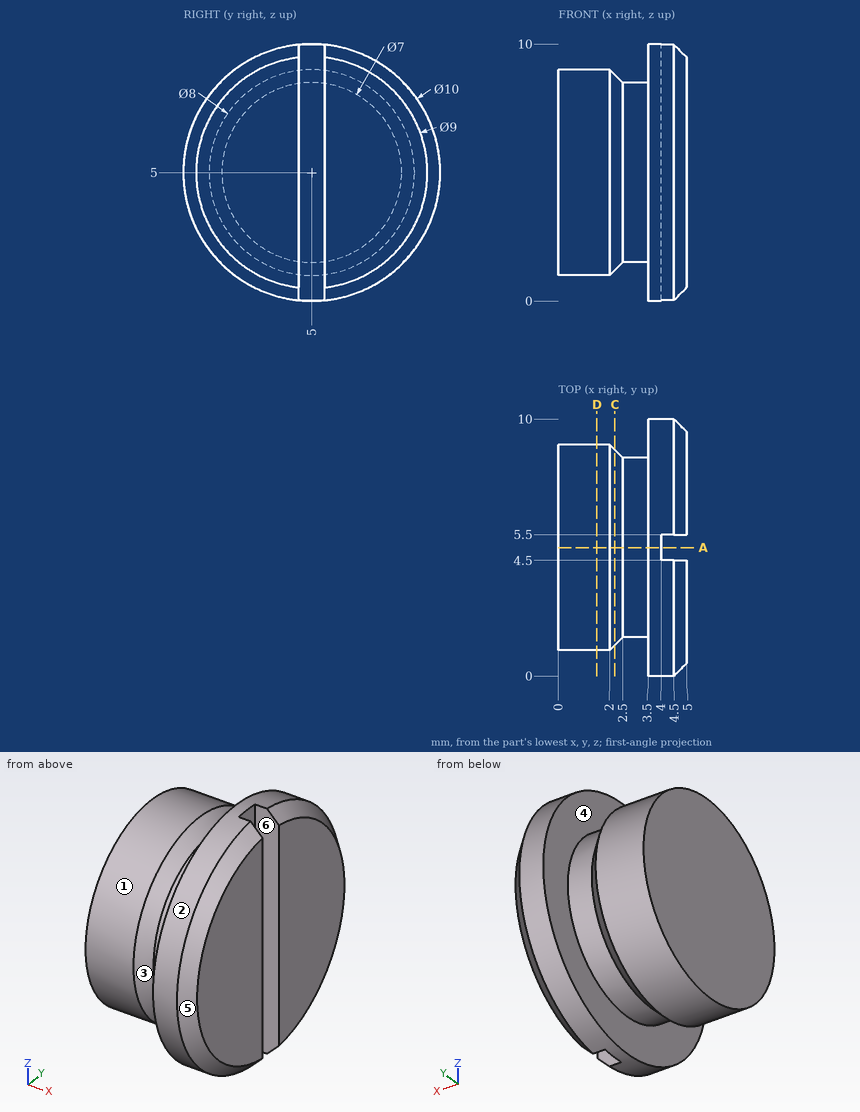
Drawing for the job (mm, zero at the part's lowest x, y, z). A direction names the side the tool comes from. Coordinates: 2 decimals unless noted, no trailing zeros. Order: outer loops, then holes, each group sorted by start corner. A loop starts at its lowest first (then second) coordinate and runs counter-clockwise, first axis right, second up. Notation, with made-up numbers: (-1.75, -33.5) -> (22.25, -33.5) arc R14 ccw to (22.25, -8.5) -> close; hole circle Ø10 at (54.5, 53.25). An arc over 180 degrees is marked (long way). Answer in a Markdown table with one row per item.
1) Band-saw the part on C-C (x = 2.2). List the corners of the cut face in (y, z), and give its area (3 significant figures).
Check values:
| item | result |
|---|---|
| outline | circle Ø7.6 at (5, 5) |
| area | 45.4 mm2 |
2) Flat gauge pins, fed straight in: P1, Ø1.1, axis at x = 4.5, z = 2.5, coming from the -Y side; P2, Ø1.5, axis at x = 2.5, z = 7.5, coming from the -Y side; P3, Ø2, axis at x = 2, y = 5, coming from the -Z side. Where does each tip first touch, or does it go through?
Check values:
| item | result |
|---|---|
| P1 | y = 0.4 |
| P2 | y = 1.5 |
| P3 | z = 1 |
3) Band-saw the part on D-D (x = 1.5). List the corners of the cut face in (y, z), and give its area (3 significant figures).
Check values:
| item | result |
|---|---|
| outline | circle Ø8 at (5, 5) |
| area | 50.3 mm2 |
4) Which spindle directions (+Z, -Z, +X, -X, +Y, -Y) get a long thin tool onto all of the face, cutting with end or side? Do the marked faces 1, 2 and 3. Say none if no direction does.
Check values:
| item | result |
|---|---|
| face 1 | -X |
| face 2 | +X, -X |
| face 3 | none |
5) Band-saw the part on A-A (y = 5). List the corners of the cut face in (x, z).
Check values:
| item | result |
|---|---|
| outline | (0, 1) -> (2, 1) -> (2.5, 1.5) -> (3.5, 1.5) -> (3.5, 0) -> (4, 0) -> (4, 10) -> (3.5, 10) -> (3.5, 8.5) -> (2.5, 8.5) -> (2, 9) -> (0, 9) -> close |
6) Drill centre lines: line 1 (X direction, y = 5, z = 6); line 2 (X direction, y = 6, z = 1.5); line 3 (X direction, y = 1.5, z = 3.5). Where is each one in solid material? Low to high.
Check values:
| item | result |
|---|---|
| line 1 | 0 to 4 |
| line 2 | 0 to 2.36, 3.5 to 5 |
| line 3 | 0 to 2.19, 3.5 to 5 |
7) Mould opens along X. For the marked faces 4, 5 and 6 say: pulls with the +X half, pulls with the -X half, needs draft (parallel to the pull), parting line crosses it, or undercut.
Check values:
| item | result |
|---|---|
| face 4 | undercut |
| face 5 | pulls with the +X half |
| face 6 | needs draft |
